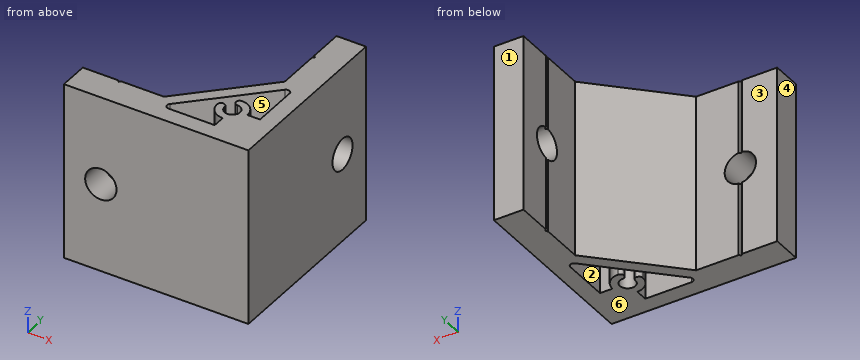
from build123d import *

# Parameters (mm, degrees)
EXTRUDE_1_DEPTH     = 24
SKETCH_2_R          = 4.25
CUT_EXTRUDE_1_DEPTH = 9
SKETCH_3_R          = 4.25
CUT_EXTRUDE_2_DEPTH = 9


with BuildPart() as part:
    # Эскиз1 → Бобышка-Вытянуть1 (new body, symmetric)
    with BuildSketch(Plane.XY):
        Polygon((-50, 0), (0, 0), (0, 50), (-8, 50), (-8, 40.5), (-7.5, 40), (-8, 39.5), (-8, 28), (-28, 8), (-39.5, 8), (-40, 7.5), (-40.5, 8), (-50, 8), align=None)
        with BuildLine():
            Line((-4.5, 12), (-4.5, 24.560303038))
            ThreePointArc((-4.5, 24.560303038), (-5.117316568, 25.484182571), (-6.207106781, 25.267409819))
            Line((-6.207106781, 25.267409819), (-25.267409819, 6.207106781))
            ThreePointArc((-25.267409819, 6.207106781), (-25.484182571, 5.117316568), (-24.560303038, 4.5))
            Line((-24.560303038, 4.5), (-12, 4.5))
            Line((-12, 4.5), (-12, 7.9))
            ThreePointArc((-12, 7.9), (-14.899137803, 9.100862197), (-16.1, 12))
            ThreePointArc((-16.1, 12), (-15.1, 13), (-14.1, 12))
            ThreePointArc((-14.1, 12), (-10.51507576, 10.51507576), (-12, 14.1))
            ThreePointArc((-12, 14.1), (-13, 15.1), (-12, 16.1))
            ThreePointArc((-12, 16.1), (-9.100862197, 14.899137803), (-7.9, 12))
            Line((-7.9, 12), (-4.5, 12))
        make_face(mode=Mode.SUBTRACT)
    extrude(amount=EXTRUDE_1_DEPTH, both=True)

    # Эскиз2 → Вырез-Вытянуть1 (cut, through all)
    with BuildSketch(Plane.ZY.offset(8)):
        with Locations(Location((0, 40, 0), (0, 0, 270))):  # turned: the seam where the file's is
            Circle(SKETCH_2_R)
    extrude(amount=-CUT_EXTRUDE_1_DEPTH, mode=Mode.SUBTRACT)

    # Эскиз3 → Вырез-Вытянуть2 (cut, through all)
    with BuildSketch(Plane(origin=(0, 8, 0), x_dir=(1, 0, 0), z_dir=(0, 1, 0))):
        with Locations(Location((-40, 0, 0), (0, 0, 180))):  # turned: the seam where the file's is
            Circle(SKETCH_3_R)
    extrude(amount=-CUT_EXTRUDE_2_DEPTH, mode=Mode.SUBTRACT)


solid = part.part
Model file for the job. Use its own axes, mm. Face numbers are marked on the shaded views. A direction names the side the tool comes from. Round coordinates to 2 decimals unless told otherwise and drop trailing zeros. Order: outer loops, then holes, each group sorted by start corner. A loop starts at its lowest first (then second) coordinate and runs counter-clockwise, first axis right, second up. Notation, with made-up numbers: M 74.25,-1.75 L 126.25,-1.75 A17 cw 126.25,28.25 Z; hole C -3.75,-0.75 d8. An arc over 180 degrees is marked long. Write each question's results on one line, items separated by ' | '. Start each with the question number.
(1) Which spindle directions (+Z, -Z, +X, -X, +Y, -Y) get a long thin tool onto all of the face, cutting with end or side? Do the marked faces 1, 2 and 3. Say none if no direction does.
(2) Saw through at C-C, the plane x = -43.5. Give the cut face in (y, z).
(3) Saw through at B-B, the plane y = 15.1. Give the cut face in (x, z).
(4) Probe probe 1 along X at (y, z) = (3, 0); probe 2 along Y at (x, z) = (-11, -18.5); probe 3 along Y at (x, z) = (-4, 0). List the from-to ranges inside material, lowest first. Write a range as from..to.
(5) Two-plate mould, pull along X, no slides. Class the marked faces 4, 5 and 6: pulls with the +X half, pulls with the -X half, needs draft (parallel to the pull), parting line crosses it, or undercut.
(6) Drop flat-ended pins along their axis: pin 1 (10 mm diameter, centred on y = 40, z = 0, fed in from -X); pin 2 (1.5 mm diameter, centred on x = -9.5, y = 43.5, fed in from -Z); pin 3 (12.5 mm diameter, centred on x = -33.5, z = -10, fed in from +Y); pin 4 (6.5 mm diameter, centred on y = 19, z = 0.5, fed in from -X). Give the stop position or say it passes through.
(7) Saw through at A-A, the plane z = 0. Give the cut face in (x, y), then the cut area to 3 significant figures.
(8) Saw through at D-D, the plane z = -5.5. Give the cut face in (x, y).
Established:
1) face 1: +Z, -Z, +X, -X, +Y | face 2: +Z, -Z | face 3: +Z, -Z, -X, +Y
2) outline: M 0,-24 L 8,-24 L 8,-2.41 L 0,-2.41 Z; M 0,2.41 L 8,2.41 L 8,24 L 0,24 Z
3) outline: M -20.9,-24 L -16.37,-24 L -16.37,24 L -20.9,24 Z; M -13,-24 L -9.32,-24 L -9.32,24 L -13,24 Z; M -4.5,-24 L 0,-24 L 0,24 L -4.5,24 Z
4) probe 1: x = -50..-44.25, -35.75..0 | probe 2: y = 0..10.15, 13.85..15.98, 20.47..25 | probe 3: y = 0..35.75, 44.25..50
5) face 4: pulls with the -X half | face 5: undercut | face 6: needs draft
6) pin 1: stops at x = -8 | pin 2: passes through | pin 3: stops at y = 8.75 | pin 4: stops at x = -20.25
7) outline: M -50,0 L -44.25,0 L -44.25,8 L -50,8 Z; M -35.75,0 L 0,0 L 0,35.75 L -8,35.75 L -8,28 L -28,8 L -35.75,8 Z; M -8,44.25 L 0,44.25 L 0,50 L -8,50 Z; hole M -25.27,6.21 A1 ccw -24.56,4.5 L -12,4.5 L -12,7.9 A4.1 cw -16.1,12 A1 cw -14.1,12 A2.1 ccw long -12,14.1 A1 cw -12,16.1 A4.1 cw -7.9,12 L -4.5,12 L -4.5,24.56 A1 ccw -6.21,25.27 Z | area: 625 mm^2
8) outline: M -50,0 L 0,0 L 0,50 L -8,50 L -8,40.5 L -7.5,40 L -8,39.5 L -8,28 L -28,8 L -39.5,8 L -40,7.5 L -40.5,8 L -50,8 Z; hole M -25.27,6.21 A1 ccw -24.56,4.5 L -12,4.5 L -12,7.9 A4.1 cw -16.1,12 A1 cw -14.1,12 A2.1 ccw long -12,14.1 A1 cw -12,16.1 A4.1 cw -7.9,12 L -4.5,12 L -4.5,24.56 A1 ccw -6.21,25.27 Z
